```python
from build123d import *

# Parameters (mm, degrees)
CYLINDER011_R     = 1.5
CYLINDER011_DEPTH = 27
ARRAY004_X_COUNT  = 2
ARRAY004_X_PITCH  = 30
ARRAY004_Y_COUNT  = 2
ARRAY004_Y_PITCH  = 23.5
ARRAY003_X_COUNT  = 3
ARRAY003_X_PITCH  = 10
ARRAY003_Y_COUNT  = 3
ARRAY003_Y_PITCH  = 10
BOX008_W          = 38
BOX008_H          = 32
BOX008_DEPTH      = 32
FILLET005_R       = 5


with BuildPart() as coaster_screw_hole:
    # Cylinder011 → Cylinder011 (new body)
    with BuildSketch(Plane.XY):
        Circle(CYLINDER011_R)
    extrude(amount=CYLINDER011_DEPTH)


with BuildPart() as coaster_holder_bottom_hole_array:
    # Array004 base: copy of coaster screw hole
    add(coaster_screw_hole.part)

    # Array004 X: coaster holder bottom hole array ×2


with BuildPart() as coaster_holder_bottom_hole_array_1:
    add(coaster_holder_bottom_hole_array.part)
    with Locations(*[(i * ARRAY004_X_PITCH, 0, 0) for i in range(1, ARRAY004_X_COUNT)]):
        add(coaster_holder_bottom_hole_array.part)

    # Array004 Y: coaster holder bottom hole array ×2


with BuildPart() as coaster_holder_bottom_hole_array_2:
    add(coaster_holder_bottom_hole_array_1.part)
    with Locations(*[(0, i * ARRAY004_Y_PITCH, 0) for i in range(1, ARRAY004_Y_COUNT)]):
        add(coaster_holder_bottom_hole_array_1.part)


with BuildPart() as coaster_holder_bottom_hole_array_3:
    # Array004 placement: moved
    add(coaster_holder_bottom_hole_array_2.part.moved(Location((-15, -11.75, 0))))


with BuildPart() as coaster_hole_fusion:
    # Array003 base: copy of coaster screw hole
    add(coaster_screw_hole.part)

    # Array003 X: coaster hole fusion ×3


with BuildPart() as coaster_hole_fusion_1:
    add(coaster_hole_fusion.part)
    with Locations(*[(i * ARRAY003_X_PITCH, 0, 0) for i in range(1, ARRAY003_X_COUNT)]):
        add(coaster_hole_fusion.part)

    # Array003 Y: coaster hole fusion ×3


with BuildPart() as coaster_hole_fusion_2:
    add(coaster_hole_fusion_1.part)
    with Locations(*[(0, i * ARRAY003_Y_PITCH, 0) for i in range(1, ARRAY003_Y_COUNT)]):
        add(coaster_hole_fusion_1.part)


with BuildPart() as coaster_hole_fusion_3:
    # Array003 placement: moved
    add(coaster_hole_fusion_2.part.moved(Location((-10, -10, 16))))

    # Fusion011: union coaster holder bottom hole array
    add(coaster_holder_bottom_hole_array_3.part)


with BuildPart() as coaster_holder_cut:
    # Box008 → Box008 (new body)
    with BuildSketch(Plane(origin=(-19, -16, 0), x_dir=(1, 0, 0), z_dir=(0, 0, 1))):
        with Locations((19, 16)):
            Rectangle(BOX008_W, BOX008_H)
    extrude(amount=BOX008_DEPTH)

    # Fillet005
    fillet005_edges = [coaster_holder_cut.edges().sort_by_distance(p)[0] for p in [
        (-19, -16, 16),
        (-19, 16, 16),
        (19, -16, 16),
        (19, 16, 16),
    ]]
    fillet(fillet005_edges, radius=FILLET005_R)

    # Cut004004: cut coaster hole fusion
    add(coaster_hole_fusion_3.part, mode=Mode.SUBTRACT)


solid = coaster_holder_cut.part
```
Can you work these out from the model? Positions are in its coordinate system, mm. A direction names the side the tool comes from. Give positions to 0.01 mm unless a question says otherwise; leave off trailing zeros. Write each loop counter-clockwise with the first axis right and the second up, starting at its lowest first coordinate (ties: lowest second). Pieces come first, ordered by that corner, then holes. Notation, with made-up numbers: (-12, 14.25) - (-6, 14.25) arc R13 cw to (-6, 32.25) - close; hole circle Ø2 at (61.25, 1). An arc over 180 degrees is marked (long way). Write item = value, one per line. Start each with the question number.
1. Imagine slicing it at A-A (z = 7.5). Please give me the cut outline in (x, y), and give its area (3 significant figures).
2. Thinking about a two-plate mould opening in X: for faces 1 (the face through (-18, -14, 16)), 2 (the face through (0, 0, 0)), 3 (the face through (17, -15, 16)), 4 (the face through (15, 12, 27)), which applies, released by +X, released by -X, zero draft, split by the parting line, or undercut?
3. Please list where these lines run through material, in increasing order: line 1 (X direction, y = 10, z = 20); line 2 (Y direction, x = 10, z = 25); line 3 (Y direction, x = 14, z = 9).
4. On a 3-axis mill with a long thin cutter (end or side, diameter ignored), from which of +Z, -Z, +X, -X, +Y, -Y can I reach the whole of each face in a straight line? I mean faces 5 (the face through (19, 0, 16)), 6 (the face through (-15, -12, 27)), 7 (the face through (-0.325, -11.464, 23.888)). Say none if no direction works.
5. Imagine slicing it at B-B (y = 0). Please give me the cut outline in (x, z).
6. Imagine slicing it at C-C (z = 23). Count the separate pieces of the cut face and the enclosed holes in it, and give its area (3 significant figures).
7. For pin 1 (0.9 mm diameter, centred on x = 15.5, y = -12.5, fed in from -Z); pin 2 (0.9 mm diameter, centred on x = -10, y = -9.5, fed in from +Z), each with a flat end and sliding along its axis, tell me the tip position at first contact or that it passes through.
8. Imagine slicing it at D-D (x = -10). Please give me the cut outline in (y, z).
Worked answers:
q1.outline = (-19, -11) arc R5 ccw to (-14, -16) - (14, -16) arc R5 ccw to (19, -11) - (19, 11) arc R5 ccw to (14, 16) - (-14, 16) arc R5 ccw to (-19, 11) - close; hole circle Ø3 at (-15, -11.75); hole circle Ø3 at (-15, 11.75); hole circle Ø3 at (15, -11.75); hole circle Ø3 at (15, 11.75)
q1.area = 1,170 mm2
q2.face_1 = released by -X
q2.face_2 = zero draft
q2.face_3 = released by +X
q2.face_4 = undercut
q3.line_1 = -19 to -11.5, -8.5 to -1.5, 1.5 to 8.5, 11.5 to 19
q3.line_2 = -16 to -11.5, -8.5 to -1.5, 1.5 to 8.5, 11.5 to 16
q3.line_3 = -16 to -12.87, -10.63 to 10.63, 12.87 to 16
q4.face_5 = +Z, -Z, +X, +Y, -Y
q4.face_6 = -Z
q4.face_7 = +Z
q5.outline = (-19, 0) - (19, 0) - (19, 32) - (11.5, 32) - (11.5, 16) - (8.5, 16) - (8.5, 32) - (1.5, 32) - (1.5, 16) - (-1.5, 16) - (-1.5, 32) - (-8.5, 32) - (-8.5, 16) - (-11.5, 16) - (-11.5, 32) - (-19, 32) - close
q6.separate_pieces = 1
q6.enclosed_holes = 13
q6.area = 1,100 mm2
q7.pin_1 = 27
q7.pin_2 = 16
q8.outline = (-16, 0) - (16, 0) - (16, 32) - (11.5, 32) - (11.5, 16) - (8.5, 16) - (8.5, 32) - (1.5, 32) - (1.5, 16) - (-1.5, 16) - (-1.5, 32) - (-8.5, 32) - (-8.5, 16) - (-11.5, 16) - (-11.5, 32) - (-16, 32) - close
